Geometry check sheet. Reference: the model listing, model coordinates, mm. Coordinates: 2 decimals unless noted, no trailing zeros. Write each loop counter-clockwise with the first axis right and the second up, starting at its lowest first coordinate (ties: lowest second). Pieces come first, ordered by that corner, then holes. Notation, with made-up numbers: (56.5, 18) -> (74.5, 18) arc R21 ccw to (74.5, 57) -> close; hole circle Ø11 at (46, 30). An arc over 180 degrees is marked (long way). Answer in a Markdown table with one row per item. Add a question column.
1. Scan lines: L1, parallel to X at y = -1074, z = 506.5; L2, parallel to X at y = -919, z = 610; L3, parallel to Y at x = 686.5, z = 61. Record each from-to range of solid material in increasing order. Write a range as from..to.
2. Mould release check, pull along Y, two halves, no side actions. Record for faces 1 (the cylindrical face through (802.61, -1143.01, 493)), 2 (the flat face through (710.421, -2141.412, 493)), 3 (the cylindrical face through (799.61, -1142.99, 493)), 4 (the flat face through (801, -1191, 1000)): pulls with the +Y half, pulls with the -Y half, needs draft (parallel to the pull), parting line crosses it, or undercut.
3. Cross-section at A-A on z = 221. Record the cut outline in (x, y).
4. Cross-section at B-B on y = -652. Record the cut outline in (x, z).
5. Depth check by flat-ended pin: P1, Ø1, axis at x = 714, z = 582.5, coming from the -Y side. Enter the tip coordinate at first touch or a pass-through.
6. Cross-section at C-C on x = 704. Record the cut outline in (y, z), and give its area (3 significant figures).
Autodesk Inventor part; units mm, degrees
ref_plane "YZ Plane" through (0, 0, 0) normal (1, 0, 0) x (0, 1, 0)
ref_plane "XZ Plane" through (0, 0, 0) normal (0, 1, 0) x (-1, 0, 0)
ref_plane "XY Plane" through (0, 0, 0) normal (0, 0, 1) x (1, 0, 0)
sketch "Sketch1" plane through (0, 0, 0) normal (0, 0, 1) x (1, 0, 0)
  line L0 (-750, 0) -> (750, 0) construction
  line L1 (750, 0) -> (750, -2700) construction
  line L2 (750, -2700) -> (-750, -2700) construction
  line L3 (-750, -2700) -> (-750, 0) construction
  line L4 (800, 50) -> (-800, 50) construction
  line L5 (-800, 50) -> (-800, -2750) construction
  line L6 (-800, -2750) -> (800, -2750) construction
  line L7 (800, -2750) -> (800, 50) construction
  line L8 (-850, 100) -> (850, 100) construction
  line L9 (850, 100) -> (850, -2800) construction
  line L10 (850, -2800) -> (-850, -2800) construction
  line L11 (-850, -2800) -> (-850, 100) construction
  arc A0 (750, 0) -> (743.691501, 0.841272) centre (0, -5600) ccw construction
  line L12 (-750, -2100) -> (750, -2100) construction
  line L13 (115.485997, -2697.8227) -> (669.21004, -2176.118213) construction
  arc A1 (750, -2100) -> (750.178737, -2098.125829) centre (-10250, -1050) ccw construction
  line L14 (750, 0) -> (749.60177, -2.973451) construction
  arc A2 (750, -3.026786) -> (0, 47) centre (-0.2, -5602.999996) ccw construction
  line L15 (750, 0) -> (747.013575, -0.285068) construction
  arc A3 (767.164125, -238.640862) -> (747.4657, -5.032602) centre (-10252.989512, -1050.252733) ccw construction
  arc A4 (750.602724, -6.333527) -> (743.691501, 0.841272) centre (742.638487, -7.089123) ccw construction
  arc A5 (747.4657, -5.032602) -> (744.874766, -2.342571) centre (744.479152, -5.316372) ccw construction
  line L16 (750, -2100) -> (752.986425, -2100.285068) construction
  arc A6 (752.986425, -2100.285068) -> (771.283058, -213.26303) centre (-10246.989147, -1050.029193) ccw construction
  line L17 (750, -2100) -> (752.057249, -2102.183512) construction
  line L18 (752.05726, -2102.183502) -> (752.057249, -2102.183512) construction
  arc A7 (748.630029, -2101.290751) -> (750.178737, -2098.125829) centre (745.201281, -2097.651564) ccw
  line L19 (0, -2697) -> (110.793766, -2697) construction
  line L20 (112.851015, -2696.183512) -> (685.348728, -2156.790959) construction
  arc A8 (110, -2700) -> (115.485997, -2697.8227) centre (110, -2692) ccw construction
  arc A9 (110.793766, -2697) -> (112.851015, -2696.183512) centre (110.793766, -2694) ccw construction
  line L21 (685.348728, -2156.790959) -> (687.405977, -2158.974471) construction
  line L22 (752.05726, -2102.183502) -> (671.267289, -2178.301725) construction
  line L23 (671.267289, -2178.301725) -> (669.21004, -2176.118213) construction
  arc A10 (747.4657, -5.032602) -> (747.013575, -0.285068) centre (-10252.989512, -1050.252733) ccw construction
  arc A11 (743.691501, 0.841272) -> (0, 50) centre (0, -5600) ccw construction
  arc A12 (750.602724, -6.333527) -> (750, 0) centre (-10250, -1050) ccw construction
  line L24 (770.156022, -238.420524) -> (767.164125, -238.640862) construction
  line L25 (768.291667, -213.490137) -> (771.283058, -213.26303) construction
  arc A13 (768.291667, -213.490137) -> (750.602724, -6.333527) centre (-10250, -1050) ccw construction
  line L26 (0, 100) -> (0, 50) construction
  line L27 (0, -2700) -> (0, -2697) construction
  line L28 (0, 47) -> (0, 0) construction
  line L29 (0, 50) -> (0, 47) construction
  arc A14 (752.057249, -2102.183512) -> (752.986425, -2100.285068) centre (749.999822, -2099.999913) ccw construction
  line L30 (669.21004, -2176.118213) -> (748.630029, -2101.290751)
  arc A15 (750.178737, -2098.125829) -> (768.291667, -213.490137) centre (-10250, -1050) ccw
  line L31 (748.630029, -2101.290751) -> (750, -2100) construction
  point P0 (0, -2750)
  dimension "d54" = 1500
  dimension "d55" = 2700
  dimension "d58" = 2100
  dimension "d68" = 8
  dimension "d70" = 3
  dimension "d75" = 5
  dimension "d83" = 8
  dimension "d86" = 3
  dimension "d112" = 239.271
  dimension "d113" = 50
  dimension "d114" = 50
  dimension "d115" = 3
  dimension "d116" = 25
  dimension "d117" = 110
  dimension "d118" = 25
  dimension "d119" = 111
contour flange "Contour Flange2" sketch "Sketch1" thickness 3 bend radius 5 width 1000 along (0, 0, 1) mid plane no both sides no wall seen from (708.920034, -2138.704482, 0) lies toward (0.6857497, -0.7278375, 0) curves L30 A7 A15
bend "Bend2"
corner "Corner2"
equation "\"d36\" = Thickness"
equation "\"d37\" = BendReliefWidth"
equation "\"d38\" = BendReliefDepth"
equation "\"d39\" = MinimumRemnant"
equation "\"d40\" = TransitionRadius"
equation "\"d42\" = BendRadius"
equation "\"d44\" = CornerReliefSize"
equation "\"d45\" = GapSize"
equation "\"d46\" = JacobiRadiusSize"
equation "\"BendReliefWidth\" = Thickness"
equation "\"BendReliefDepth\" = 0.5 * Thickness"
equation "\"CornerReliefSize\" = 4 * Thickness"
equation "\"MinimumRemnant\" = 2 * Thickness"
equation "\"GapSize\" = Thickness"
properties part number "МОО 024 лист борт основной" material "Stainless Steel AISI 304"
Results found:
| question | item | result |
|---|---|---|
| 1 | L1 | x = 799.97..802.97 |
| 1 | L2 | x = 799.22..802.22 |
| 1 | L3 | y = -2163.95..-2159.83 |
| 2 | face 1 | parting line crosses it |
| 2 | face 2 | pulls with the -Y half |
| 2 | face 3 | undercut |
| 2 | face 4 | needs draft |
| 3 | outline | (669.21, -2176.12) -> (671.27, -2178.3) -> (750.69, -2103.47) arc R8 ccw to (753.17, -2098.41) arc R11053 ccw to (771.28, -213.26) -> (768.29, -213.49) arc R11050 cw to (750.18, -2098.13) arc R5 cw to (748.63, -2101.29) -> close |
| 4 | outline | (792.83, 0) -> (795.83, 0) -> (795.83, 1000) -> (792.83, 1000) -> close |
| 5 | P1 | stops at y = -2138.51 |
| 6 | outline | (-2147.46, 0) -> (-2143.34, 0) -> (-2143.34, 1000) -> (-2147.46, 1000) -> close |
| 6 | area | 4,120 mm^2 |
